The model under review builds one solid part; all positions refer to its coordinate system, in mm. Coordinates: 2 decimals unless noted, no trailing zeros. Order: outer loops, then holes, each group sorted by start corner. A loop starts at its lowest first (then second) coordinate and runs counter-clockwise, first axis right, second up.
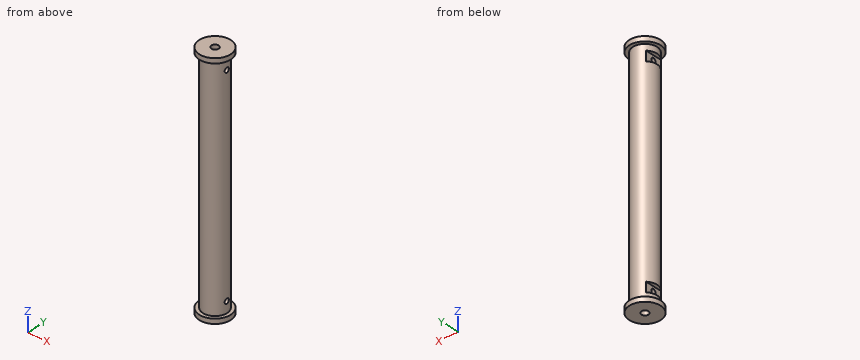
from build123d import *

# Parameters (mm, degrees)
SKETCH1_R                       = 10
SKETCH1_R_2                     = 3
BOSS_EXTRUDE1_DEPTH             = 199
SKETCH2_R                       = 13
SKETCH2_R_2                     = 10
BOSS_EXTRUDE2_DEPTH             = 4
CUT_EXTRUDE1_START              = -25
SKETCH3_W                       = 3
SKETCH3_H                       = 8
CUT_EXTRUDE1_DEPTH              = 47
F_4_0MM_CLEARANCE_DOWEL_HOLE1_D = 4


with BuildPart() as part:
    # Sketch1 → Boss-Extrude1 (new body)
    with BuildSketch(Plane.XY):
        Circle(SKETCH1_R)
        Circle(SKETCH1_R_2, mode=Mode.SUBTRACT)
    extrude(amount=BOSS_EXTRUDE1_DEPTH)

    # Sketch2 → Boss-Extrude2 (add)
    with BuildSketch(Plane(origin=(0, 0, 0), x_dir=(-1, 0, 0), z_dir=(0, 0, -1))):
        Circle(SKETCH2_R)
        Circle(SKETCH2_R_2, mode=Mode.SUBTRACT)
    boss_extrude2 = extrude(amount=-BOSS_EXTRUDE2_DEPTH)

    # Mirror1: Boss-Extrude2 across plane
    add(boss_extrude2.mirror(Plane(origin=(0, 0, 99.5), x_dir=(1, 0, 0), z_dir=(0, 0, -1))))

    # Sketch3 → Cut-Extrude1 (cut)
    with BuildSketch(Plane(origin=(0, 0, 0), x_dir=(1, 0, 0), z_dir=(0, 1, 0)).offset(CUT_EXTRUDE1_START)):
        with Locations((-8.5, -186)):
            Rectangle(SKETCH3_W, SKETCH3_H)
    cut_extrude1 = extrude(amount=CUT_EXTRUDE1_DEPTH, mode=Mode.SUBTRACT)

    # Ø4.0mm Clearance Dowel Hole1 (through all)
    with Locations(Plane(origin=(-7, 0, 186), x_dir=(0, 0, -1), z_dir=(-1, 0, 0))):
        with Locations((0, 0)):
            f_4_0mm_clearance_dowel_hole1 = Hole(F_4_0MM_CLEARANCE_DOWEL_HOLE1_D / 2)

    # Mirror2: Cut-Extrude1, Ø4.0mm Clearance Dowel Hole1 across plane
    add(cut_extrude1.mirror(Plane(origin=(0, 0, 99.5), x_dir=(1, 0, 0), z_dir=(0, 0, -1))), mode=Mode.SUBTRACT)
    add(f_4_0mm_clearance_dowel_hole1.mirror(Plane(origin=(0, 0, 99.5), x_dir=(1, 0, 0), z_dir=(0, 0, -1))), mode=Mode.SUBTRACT)


solid = part.part
(1) Consider section A-A (x = 0). Give the boundary of the cut face in (y, z).
(2) Consider section D-D (z = 13). Give the boundary of the cut face in (x, y).
(3) Consider section C-C (x = 7.5). Give the boundary of the cut face in (y, z).
(4) Wall thickness on line 1 (Y direction, x = 0, z = 176); line 2 (Z direction, x = -2.5, y = 11.5): over which ranges is each line inside the solid? List them lowest first.
(5) Consider section B-B (y = 0). Give the number of separate pieces and of enclosed holes in the cut face, then the cut area to 3 significant figures.
(6) Insertion check: pin 1 Ø12 at (y, z) = (6.5, 62.5) entering from +X; pin 2 Ø3.5 at (x, y) = (-9, -2.5) entering from -Z; pin 3 Ø4.5 at (y, z) = (0, 13) entering from -X; pin 4 Ø4 at (x, z) = (-3, 100.5) entering from +Y. Each pin has a flat end and moves straight along its axis. Give the tip position at first contact, or say it passes through.
Findings:
1. outline: (-13, 0) - (-3, 0) - (-3, 199) - (-13, 199) - (-13, 195) - (-10, 195) - (-10, 4) - (-13, 4) - close; (3, 0) - (13, 0) - (13, 4) - (10, 4) - (10, 195) - (13, 195) - (13, 199) - (3, 199) - close
2. outline: (-7, -7.14) arc R10 ccw to (9.8, -2) - (2.24, -2) arc R3 cw to (-2.24, -2) - (-7, -2) - close; (-7, 2) - (-2.24, 2) arc R3 cw to (2.24, 2) - (9.8, 2) arc R10 ccw to (-7, 7.14) - close
3. outline: (-10.62, 0) - (10.62, 0) - (10.62, 4) - (6.61, 4) - (6.61, 195) - (10.62, 195) - (10.62, 199) - (-10.62, 199) - (-10.62, 195) - (-6.61, 195) - (-6.61, 4) - (-10.62, 4) - close; hole circle Ø4 at (0, 13); hole circle Ø4 at (0, 186)
4. line 1: y = -10 to -3, 3 to 10
4. line 2: z = 0 to 4, 195 to 199
5. separate pieces: 6
5. enclosed holes: 0
5. area: 2,700 mm2
6. pin 1: stops at x = 9.99
6. pin 2: stops at z = 0
6. pin 3: stops at x = -7
6. pin 4: stops at y = 9.95
